```python
from build123d import *

# Parameters (mm, degrees)
ESQUISSE1_R             = 2.3500000000000014
ESQUISSE1_R_2           = 2.3499999999999983
ESQUISSE1_R_3           = 2.349999999999996
BOSS_EXTRU_1_DEPTH      = 5
BOSS_EXTRU_2_DEPTH      = 8
CONG_3_R                = 2
CONG_4_R                = 20
ESQUISSE4_R             = 2.0000000000000036
ENL_V_MAT_EXTRU_1_DEPTH = 114.86737128447481
CONG_5_R                = 20
ENL_V_MAT_EXTRU_2_DEPTH = 114.40537131563231
BOSS_EXTRU_3_DEPTH      = 5
CONG_6_R                = 20
CONG_7_R                = 20
ESQUISSE7_R             = 2.000000000000001
ENL_V_MAT_EXTRU_3_DEPTH = 10


with BuildPart() as part:
    # Esquisse1 → Boss.-Extru.1 (new body)
    with BuildSketch(Plane(origin=(0, 0, 0), x_dir=(1, 0, 0), z_dir=(0, 1, 0))):
        Polygon((39.99999999999999, -95.00000000000003), (-40, -95.00000000000001), (-61.41480475615327, -67.3159587983287), (-40, -33.41030108504288), (-40, 33.41030108504288), (-61.41480475615327, 67.31595879832868), (-39.99999999999999, 95.00000000000001), (39.99999999999999, 95.00000000000003), (61.414804756153316, 67.31595879832868), (40.000000000000014, 33.41030108504289), (40.000000000000014, -33.41030108504289), (61.414804756153316, -67.31595879832868), align=None)
        with Locations(Location((18.009715939773823, 87.47156012506183, 0), (0, 0, 270))):
            Circle(ESQUISSE1_R, mode=Mode.SUBTRACT)
        with Locations(Location((45.96329382727553, 77.48820598648535, 0), (0, 0, 270))):
            Circle(ESQUISSE1_R_2, mode=Mode.SUBTRACT)
        with Locations(Location((41.871926953773496, 56.623628500342335, 0), (0, 0, 270))):
            Circle(ESQUISSE1_R_3, mode=Mode.SUBTRACT)
        with Locations(Location((-41.871926953773496, 56.623628500342335, 0), (0, 0, 90))):
            Circle(ESQUISSE1_R_3, mode=Mode.SUBTRACT)
        with Locations(Location((-45.96329382727553, 77.48820598648535, 0), (0, 0, 90))):
            Circle(ESQUISSE1_R_2, mode=Mode.SUBTRACT)
        with Locations(Location((-18.009715939773823, 87.47156012506183, 0), (0, 0, 90))):
            Circle(ESQUISSE1_R, mode=Mode.SUBTRACT)
        with Locations(Location((41.871926953773496, -56.623628500342335, 0), (0, 0, 90))):
            Circle(ESQUISSE1_R_3, mode=Mode.SUBTRACT)
        with Locations(Location((45.963293827275415, -77.48820598648535, 0), (0, 0, 90))):
            Circle(ESQUISSE1_R_2, mode=Mode.SUBTRACT)
        with Locations(Location((18.00971593977377, -87.47156012506183, 0), (0, 0, 90))):
            Circle(ESQUISSE1_R, mode=Mode.SUBTRACT)
        with Locations(Location((-18.00971593977388, -87.47156012506183, 0), (0, 0, 270))):
            Circle(ESQUISSE1_R, mode=Mode.SUBTRACT)
        with Locations(Location((-45.96329382727556, -77.48820598648535, 0), (0, 0, 270))):
            Circle(ESQUISSE1_R_2, mode=Mode.SUBTRACT)
        with Locations(Location((-41.871926953773496, -56.623628500342335, 0), (0, 0, 270))):
            Circle(ESQUISSE1_R_3, mode=Mode.SUBTRACT)
    extrude(amount=BOSS_EXTRU_1_DEPTH)

    # Esquisse3 → Boss.-Extru.2 (add)
    with BuildSketch(Plane(origin=(0, 5, 0), x_dir=(1, 0, 0), z_dir=(0, 1, 0))):
        Polygon((40.000000000000014, -33.41030108504289), (40.000000000000014, 33.41030108504289), (44.27204448885784, 40.174148798084595), (40.89012063233698, 42.31017104251351), (36.00000000000002, 34.567734993029916), (36.00000000000003, -34.56773499302995), (40.89012063233698, -42.31017104251351), (44.27204448885783, -40.174148798084595), align=None)
        Polygon((-40.89012063233699, -42.31017104251351), (-36.00000000000003, -34.56773499302995), (-36.00000000000002, 34.567734993029916), (-40.89012063233698, 42.31017104251351), (-44.272044488857844, 40.174148798084595), (-40.000000000000014, 33.41030108504289), (-40.000000000000014, -33.41030108504289), (-44.27204448885783, -40.174148798084595), align=None)
    extrude(amount=BOSS_EXTRU_2_DEPTH)

    # Congé3
    cong_3_edges = [part.edges().sort_by_distance(p)[0] for p in [
        (-40.89012063233698, 9, -42.31017104251351),
        (-44.272044488857844, 9, -40.174148798084595),
        (-44.27204448885783, 9, 40.174148798084595),
        (-40.89012063233699, 9, 42.31017104251351),
        (40.89012063233698, 9, 42.31017104251351),
        (44.27204448885783, 9, 40.174148798084595),
        (40.89012063233698, 9, -42.31017104251351),
        (44.27204448885784, 9, -40.174148798084595),
    ]]
    fillet(cong_3_edges, radius=CONG_3_R - 0.0001)  # a hair under: the kernel refuses the full size

    # Congé4
    cong_4_edges = [part.edges().sort_by_distance(p)[0] for p in [
        (-40.00000000000001, 6.5, 33.41030108504289),
        (-40.00000000000001, 6.5, -33.41030108504289),
        (40.000000000000014, 6.5, -33.41030108504289),
        (40.000000000000014, 6.5, 33.41030108504289),
    ]]
    fillet(cong_4_edges, radius=CONG_4_R)

    # Esquisse4 → Enlèv. mat.-Extru.1 (cut, through all)
    with BuildSketch(Plane(origin=(0, 0, 0), x_dir=(-1, 0, 0), z_dir=(0, -1, 0))):
        with Locations(Location((32.99999999999999, -38.000000000000014, 0), (0, 0, 90))):
            Circle(ESQUISSE4_R)
        with Locations(Location((33.00000000000002, 38, 0), (0, 0, 90))):
            Circle(ESQUISSE4_R)
        with Locations(Location((-32.99999999999999, -38.000000000000014, 0), (0, 0, 90))):
            Circle(ESQUISSE4_R)
        with Locations(Location((-33.00000000000002, 38, 0), (0, 0, 90))):
            Circle(ESQUISSE4_R)
    extrude(amount=-ENL_V_MAT_EXTRU_1_DEPTH, mode=Mode.SUBTRACT)

    # Congé5
    cong_5_edges = [part.edges().sort_by_distance(p)[0] for p in [
        (-36.00000000000003, 9, 34.56773499302995),
        (-36.00000000000002, 9, -34.567734993029916),
        (36.00000000000002, 9, -34.567734993029916),
        (36.00000000000003, 9, 34.56773499302995),
    ]]
    fillet(cong_5_edges, radius=CONG_5_R)

    # Esquisse5 → Enlèv. mat.-Extru.2 (cut, through all)
    with BuildSketch(Plane(origin=(0, 5, 0), x_dir=(1, 0, 0), z_dir=(0, 1, 0))):
        with BuildLine():
            Line((-19, -65), (-19.00000000000001, -15))
            ThreePointArc((-19.00000000000001, -15), (-15.000000000000002, -10.999999999999979), (-10.999999999999988, -15.000000000000014))
            Line((-10.999999999999988, -15.000000000000014), (-10.999999999999979, -64.99999999999999))
            ThreePointArc((-10.999999999999979, -64.99999999999999), (-14.999999999999993, -69), (-19, -65))
        make_face()
        with BuildLine():
            Line((19.00000000000002, -64.99999999999999), (19.00000000000001, -15))
            ThreePointArc((19.00000000000001, -15), (15.000000000000005, -10.999999999999961), (10.99999999999997, -15.000000000000007))
            Line((10.99999999999997, -15.000000000000007), (10.999999999999979, -64.99999999999999))
            ThreePointArc((10.999999999999979, -64.99999999999999), (15.000000000000016, -68.99999999999999), (19.00000000000002, -64.99999999999999))
        make_face()
        with BuildLine():
            Line((19.00000000000002, 64.99999999999999), (19.00000000000001, 15))
            ThreePointArc((19.00000000000001, 15), (15.000000000000009, 10.99999999999998), (10.99999999999999, 15))
            Line((10.99999999999999, 15), (10.999999999999979, 64.99999999999999))
            ThreePointArc((10.999999999999979, 64.99999999999999), (15.000000000000016, 68.99999999999999), (19.00000000000002, 64.99999999999999))
        make_face()
        with BuildLine():
            Line((-19.00000000000002, 64.99999999999999), (-19.00000000000001, 15))
            ThreePointArc((-19.00000000000001, 15), (-15.000000000000009, 10.99999999999998), (-10.99999999999999, 15))
            Line((-10.99999999999999, 15), (-10.999999999999979, 64.99999999999999))
            ThreePointArc((-10.999999999999979, 64.99999999999999), (-15.000000000000016, 68.99999999999999), (-19.00000000000002, 64.99999999999999))
        make_face()
        with BuildLine():
            Line((-4, -64.99999999999999), (-4, -15))
            ThreePointArc((-4, -15), (2.4e-16, -11), (4, -15))
            Line((4, -15), (4, -64.99999999999999))
            ThreePointArc((4, -64.99999999999999), (-7.3e-16, -68.99999999999999), (-4, -64.99999999999999))
        make_face()
        with BuildLine():
            Line((-4, 64.99999999999999), (-4, 15))
            ThreePointArc((-4, 15), (2.4e-16, 11), (4, 15))
            Line((4, 15), (4, 64.99999999999999))
            ThreePointArc((4, 64.99999999999999), (2.4e-16, 68.99999999999999), (-4, 64.99999999999999))
        make_face()
    extrude(amount=-ENL_V_MAT_EXTRU_2_DEPTH, mode=Mode.SUBTRACT)

    # Esquisse6 → Boss.-Extru.3 (add)
    with BuildSketch(Plane(origin=(0, 5, 0), x_dir=(1, 0, 0), z_dir=(0, 1, 0))):
        Polygon((-61.41480475615327, 67.31595879832868), (-57.03518322417293, 86.05279191485651), (-39.99999999999999, 95.00000000000001), align=None)
        Polygon((57.03518322417293, 86.05279191485651), (39.99999999999999, 95.00000000000001), (61.41480475615327, 67.31595879832868), align=None)
        Polygon((61.41480475615317, -67.31595879832868), (57.03518322417293, -86.05279191485651), (39.999999999999886, -95.00000000000001), align=None)
        Polygon((-57.03518322417293, -86.05279191485651), (-40.00000000000002, -95.00000000000001), (-61.4148047561533, -67.31595879832868), align=None)
    extrude(amount=-BOSS_EXTRU_3_DEPTH)

    # Congé6
    cong_6_edges = [part.edges().sort_by_distance(p)[0] for p in [
        (-57.03518322417293, 2.5, -86.05279191485651),
        (57.03518322417293, 2.5, -86.05279191485651),
        (57.03518322417293, 2.5, 86.05279191485651),
        (-57.03518322417293, 2.5, 86.05279191485651),
    ]]
    fillet(cong_6_edges, radius=CONG_6_R)

    # Congé7
    cong_7_edges = [part.edges().sort_by_distance(p)[0] for p in [
        (-40, 2.5, 95.00000000000001),
        (-61.41480475615327, 2.5, 67.3159587983287),
        (39.99999999999999, 2.5, 95.00000000000003),
        (61.414804756153316, 2.5, 67.31595879832868),
        (61.414804756153316, 2.5, -67.31595879832868),
        (39.99999999999999, 2.5, -95.00000000000003),
        (-61.41480475615327, 2.5, -67.31595879832868),
        (-39.99999999999999, 2.5, -95.00000000000001),
    ]]
    fillet(cong_7_edges, radius=CONG_7_R)

    # Esquisse7 → Enlèv. mat.-Extru.3 (cut)
    with BuildSketch(Plane(origin=(0, 0, 0), x_dir=(-1, 0, 0), z_dir=(0, -1, 0))):
        with Locations(Location((3.47e-15, 86.99999999999997, 0), (0, 0, 90))):
            Circle(ESQUISSE7_R)
    extrude(amount=-ENL_V_MAT_EXTRU_3_DEPTH, mode=Mode.SUBTRACT)


solid = part.part
```
Design review of the part built by this model. Coordinates are the model's own, in mm. A direction names the side the tool comes from. Give positions to 0.01 mm unless a question says otherwise; leave off trailing zeros. Loops run counter-clockwise (first coordinate to the right, second up) from the corner with the lowest first, then second, coordinate; pieces in that order, holes last. Notation, with made-up numbers: (47.5, 1.25) -> (68.5, 1.25) arc R9 cw to (68.5, 7.25) -> close; hole circle Ø11 at (88, 10). An arc over 180 degrees is marked (long way). Write each question's results on one line, items separated by ' | '.
Q1. Take a section at D-D, the plane z = -87. Write out the cut boundary in (x, y).
Reply:
outline: (-53.52, 0) -> (-20.31, 0) -> (-20.31, 5) -> (-53.52, 5) -> close; (-15.71, 0) -> (-2, 0) -> (-2, 5) -> (-15.71, 5) -> close; (2, 0) -> (15.71, 0) -> (15.71, 5) -> (2, 5) -> close; (20.31, 0) -> (53.52, 0) -> (53.52, 5) -> (20.31, 5) -> close
Q2. The part is to be moulded in two halves that separate along Z. For faces 5 (the face through (39, 13, -1)), 6 (the face through (36.766, 9.056, 34.264)), 7 (the face through (19.6, 2.5, -89.2)), say which applies: +Z half, -Z half, draft (parallel to the pull), parting line (faces both ways), or undercut.
Reply:
face 5: draft | face 6: +Z half | face 7: undercut
Q3. For pin 1 Ø5.5 at (y, z) = (3.5, -42) entering from -X; pin 2 Ø5.5 at (x, z) = (-18.01, 87.47) entering from +Y; pin 3 Ø4 at (y, z) = (7, 30.5) entering from +X; pin 4 Ø4 at (x, z) = (41.87, -56.62) entering from +Y, all flat-tipped, find the tip position at first contact; note any pin that passes through.
Reply:
pin 1: stops at x = -47.16 | pin 2: stops at y = 5 | pin 3: stops at x = 40.6 | pin 4: passes through
Q4. Take a section at B-B, the plane x = 0. Write out the cut boundary in (y, z), plus the area to 3 significant figures.
Reply:
outline: (0, -95) -> (5, -95) -> (5, -89) -> (0, -89) -> close; (0, -85) -> (5, -85) -> (5, -69) -> (0, -69) -> close; (0, -11) -> (5, -11) -> (5, 11) -> (0, 11) -> close; (0, 69) -> (5, 69) -> (5, 95) -> (0, 95) -> close | area: 350 mm²
Q5. Machinability: for faces 1 (the face through (-46.686, 2.535, 91.488)), 2 (the face through (40.766, 6.591, -33.106)), 3 (the face through (0, 3, -69)), 4 (the face through (-49.92, 2.08, -49.12)), which of the approach directions +Z, -Z, +X, -X, +Y, -Y give a long, thin tool a straight path to every point of the face, cutting with its end or side? Answer none if there is none.
Reply:
face 1: +Z, -X, +Y, -Y | face 2: +X, +Y, -Y | face 3: +Y, -Y | face 4: -X, +Y, -Y
Q6. Wall thickness on L1, parallel to X at y = 1.5, z = -38; L2, parallel to X at y = 6.25, z = -8; L3, parallel to X at y = 2, z = -6.5: over which ranges is each line inside the solid? List them lowest first.
Reply:
L1: x = -42.9 to -35, -31 to -19, -11 to -4, 4 to 11, 19 to 31, 35 to 42.9 | L2: x = -40 to -36, 36 to 40 | L3: x = -40 to 40
Q7. Take a section at A-A, the plane z = -17. Write out the cut boundary in (x, y), plus the area to 3 significant figures.
Reply:
outline: (-40, 0) -> (-19, 0) -> (-19, 5) -> (-36, 5) -> (-36, 13) -> (-40, 13) -> close; (-11, 0) -> (-4, 0) -> (-4, 5) -> (-11, 5) -> close; (4, 0) -> (11, 0) -> (11, 5) -> (4, 5) -> close; (19, 0) -> (40, 0) -> (40, 13) -> (36, 13) -> (36, 5) -> (19, 5) -> close | area: 344 mm²
